The listing builds one solid part. Answer for the finished solid, in the listing's coordinates (mm). Round coordinates to 2 decimals unless told otherwise and drop trailing zeros. Loops run counter-clockwise (first coordinate to the right, second up) from the corner with the lowest first, then second, coordinate; pieces in that order, holes last. Notation, with made-up numbers: (84.5, -32) - (139.5, -32) arc R12 cw to (139.5, -10) - close; hole circle Ø9 at (-3.5, 87). An arc over 180 degrees is marked (long way). One line per item, written item: value.
Autodesk Inventor part; units mm, degrees
ref_plane "Start Plane" through (0, 0, -13.0022) normal (0, 0, 1) x (1, 0, 0)
ref_plane "End Plane" through (0, 0, 240.8579) normal (0, 0, 1) x (1, 0, 0)
ref_plane "Work Plane4" through (-6.5271, 6.9371, 237.0539) normal (0.476, -0.5059, 0.7193) x (0.8682, 0.1401, -0.476)
ref_plane "Start Plane" through (0, 0, -13.0022) normal (0, 0, 1) x (1, 0, 0)
ref_plane "End Plane" through (0, 0, 240.8579) normal (0, 0, 1) x (1, 0, 0)
sketch "Sketch" plane through (0, 0, 0) normal (0, 0, 1) x (1, 0, 0)
  circle A0 centre (0, 0) radius 9.525
  dimension "d0" = 19.05
extrude "Body" add sketch "Sketch" along normal up to surface (253.86 mm away) from surface at -13.0022
sketch "Sketch2" plane through (0, 0, 0) normal (0, 0, 1) x (1, 0, 0)
  line L0 (0, 0) -> (10, 0)
ref_plane "Work Plane3" through (0, 0, 0) normal (0, -1, 0) x (1, 0, 0)
ref_plane "Work Plane4" through (-6.5271, 6.9371, 237.0539) normal (0.476, -0.5059, 0.7193) x (0.8682, 0.1401, -0.476)
split "Split1" plane through (-6.5271, 6.9371, 237.0539) removes the side toward (0.476, -0.5059, 0.7193)
ref_plane "Work Plane5" through (-6.5271, 6.9371, -9.1982) normal (0.476, -0.5059, -0.7193) x (0.1926, 0.8581, -0.476)
split "Split2" plane through (-6.5271, 6.9371, -9.1982) removes the side toward (0.476, -0.5059, -0.7193)
sketch "Sketch3" plane through (0, 0, 0) normal (0, -1, 0) x (1, 0, 0)
  line L0 (-2, -13.0022) -> (12, -13.0022)
  line L1 (-2, 240.8579) -> (12, 240.8579)
  dimension "d7" = 253.86
equation "\"d0\" = Diam"
equation "\"d1\" = G_L"
equation "\"Diam\" = 19.05"
equation "\"G_L\" = 246.25206"
equation "\"G_OFFSET_START\" = 13.00217"
equation "\"G_OFFSET_END\" = 13.00217"
equation "\"d4\" = -G_OFFSET_START"
equation "\"d5\" = G_OFFSET_END + B_L"
equation "\"B_L\" = 227.85569"
properties part number "ANSI/AISC Rolled Steel - 3/4-9.695, RB" material "Steel, Mild"
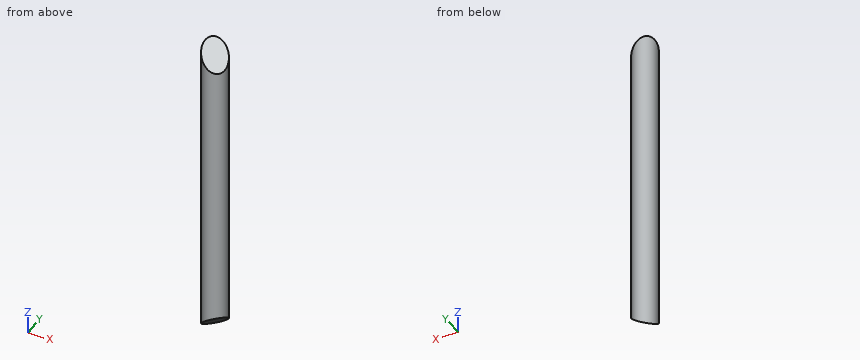
1) Consider L1, parallel to Y at x = -2.5, z = 101; L2, parallel to Z at x = -5.5, y = -7; L3, parallel to Y at x = 5.25, z = 142.5. Determine where each line is inside the solid, lowest interval first.
Final values:
L1: -9.19 to 9.19
L2: 1.28 to 226.57
L3: -7.95 to 7.95
2) A cutting plane is placed at B-B on y = -6. Give the vertices of the cut face in (x, z).
Final values:
outline: (-7.4, -0.68) - (7.4, 9.12) - (7.4, 218.74) - (-7.4, 228.53) - close
3) A cutting plane is placed at C-C on x = -5. Give the vertices of the cut face in (y, z).
Final values:
outline: (-8.11, 2.39) - (8.11, -9.01) - (8.11, 236.87) - (-8.11, 225.46) - close
4) A cutting plane is placed at A-A on z = 192. Give the vertices of the cut face in (x, y) (3 decimals).
Final values:
outline: circle Ø19.05 at (0, 0)
5) Each of these flat-tipped pins is pushed along its axis until it touches: pin 1 Ø8 at (y, z) = (-7, 117) entering from -X; pin 2 Ø1.5 at (x, y) = (2.5, -4.5) entering from -Z; pin 3 Ø3 at (x, z) = (2, 81) entering from +Y; pin 4 Ø4 at (y, z) = (-0.5, 46) entering from +X (3 decimals). Where does it stop, or does it pass through?
Final values:
pin 1: x = -9.04
pin 2: z = 4.1
pin 3: y = 9.51
pin 4: x = 9.525
